Here's how the part is built. I have some questions about the finished solid (model axes, mm). A direction names the side the tool comes from. Round coordinates to 2 decimals unless told otherwise and drop trailing zeros. Loops run counter-clockwise (first coordinate to the right, second up) from the corner with the lowest first, then second, coordinate; pieces in that order, holes last. Notation, with made-up numbers: M -38,56 L 2,56 A10 cw 2,73 Z; hole C 19.5,79 d1. An arc over 180 degrees is marked long. Answer as CSV lines item,"result".
```python
from build123d import *

# Parameters (mm, degrees)
SKETCH_1_R          = 5.75
EXTRUDE_1_DEPTH     = 0.9
SKETCH_2_R          = 5.75
SKETCH_2_R_2        = 4.8
EXTRUDE_2_DEPTH     = 3.5
SKETCH_3_R          = 6.4
SKETCH_3_R_2        = 4.8
EXTRUDE_3_DEPTH     = 1.3
SKETCH_4_W          = 0.85
SKETCH_4_H          = 3.8
SKETCH_4_W_2        = 1.824882422
SKETCH_4_H_2        = 0.85
EXTRUDE_4_DEPTH     = 6.7
EXTRUDE_5_DEPTH     = 3.8
CUT_EXTRUDE_1_REACH = 10.3
EXTRUDE_6_DEPTH     = 4
FILLET1_R           = 0.2


with BuildPart() as part:
    # Эскиз1 → Бобышка-Вытянуть1 (new body)
    with BuildSketch(Plane(origin=(0, 0, 0), x_dir=(1, 0, 0), z_dir=(0, 1, 0))):
        Circle(SKETCH_1_R)
    extrude(amount=EXTRUDE_1_DEPTH)

    # Эскиз2 → Бобышка-Вытянуть2 (add)
    with BuildSketch(Plane(origin=(0, 0.9, 0), x_dir=(1, 0, 0), z_dir=(0, 1, 0))):
        Circle(SKETCH_2_R)
        Circle(SKETCH_2_R_2, mode=Mode.SUBTRACT)
    extrude(amount=EXTRUDE_2_DEPTH)

    # Эскиз3 → Бобышка-Вытянуть3 (add)
    with BuildSketch(Plane(origin=(0, 4.4, 0), x_dir=(1, 0, 0), z_dir=(0, 1, 0))):
        Circle(SKETCH_3_R)
        Circle(SKETCH_3_R_2, mode=Mode.SUBTRACT)
    extrude(amount=EXTRUDE_3_DEPTH)

    # Эскиз4 → Бобышка-Вытянуть4 (add)
    with BuildSketch(Plane(origin=(0, 0.9, 0), x_dir=(1, 0, 0), z_dir=(0, 1, 0))):
        with Locations((-2.325, 0)):
            Rectangle(SKETCH_4_W, SKETCH_4_H)
        with Locations((2.325, 0)):
            Rectangle(SKETCH_4_W, SKETCH_4_H)
        with Locations((0, 2.325)):
            Rectangle(SKETCH_4_W_2, SKETCH_4_H_2)
        with Locations((0, -2.325)):
            Rectangle(SKETCH_4_W_2, SKETCH_4_H_2)
    extrude(amount=EXTRUDE_4_DEPTH)

    # Эскиз5 → Бобышка-Вытянуть5 (add)
    with BuildSketch(Plane(origin=(0, 0, -1.9), x_dir=(-1, 0, 0), z_dir=(0, 0, -1))):
        Polygon((1.9, 6.3), (1.6, 6.6), (2.6, 7.6), align=None)
        Polygon((-1.9, 6.3), (-1.6, 6.6), (-2.6, 7.6), align=None)
    extrude(amount=-EXTRUDE_5_DEPTH)

    # Эскиз6 → Вырез-Вытянуть1 (cut, up to next)
    with BuildSketch(Plane(origin=(0, 0, -1.9), x_dir=(-1, 0, 0), z_dir=(0, 0, -1)), mode=Mode.PRIVATE) as cut_extrude_1_sk1:
        Polygon((1.9, 6.9), (2.6, 7.6), (1.9, 7.6), align=None)
    cut_extrude_1_tool1 = extrude(cut_extrude_1_sk1.sketch, amount=-CUT_EXTRUDE_1_REACH, mode=Mode.PRIVATE) & part.part
    add(cut_extrude_1_tool1.solids().sort_by_distance((-2.133333, 7.366667, -1.9))[0], mode=Mode.SUBTRACT)
    # Эскиз6 → Вырез-Вытянуть1 (cut, up to next)
    with BuildSketch(Plane(origin=(0, 0, -1.9), x_dir=(-1, 0, 0), z_dir=(0, 0, -1)), mode=Mode.PRIVATE) as cut_extrude_1_sk2:
        Polygon((-1.9, 6.9), (-2.6, 7.6), (-1.9, 7.6), align=None)
    cut_extrude_1_tool2 = extrude(cut_extrude_1_sk2.sketch, amount=-CUT_EXTRUDE_1_REACH, mode=Mode.PRIVATE) & part.part
    add(cut_extrude_1_tool2.solids().sort_by_distance((2.133333, 7.366667, -1.9))[0], mode=Mode.SUBTRACT)

    # Эскиз7 → Бобышка-Вытянуть6 (add)
    with BuildSketch(Plane(origin=(0, 0.9, 0), x_dir=(1, 0, 0), z_dir=(0, 1, 0))):
        with BuildLine():
            Line((-0.35, -2.75), (0.35, -2.75))
            Line((0.35, -2.75), (0.35, -4.787222577))
            ThreePointArc((0.35, -4.787222577), (0, -4.8), (-0.35, -4.787222577))
            Line((-0.35, -4.787222577), (-0.35, -2.75))
        make_face()
        with BuildLine():
            Line((4.787222577, -0.35), (2.75, -0.35))
            Line((2.75, -0.35), (2.75, 0.35))
            Line((2.75, 0.35), (4.787222577, 0.35))
            ThreePointArc((4.787222577, 0.35), (4.8, 0), (4.787222577, -0.35))
        make_face()
        with BuildLine():
            Line((0.35, 2.75), (0.35, 4.787222577))
            ThreePointArc((0.35, 4.787222577), (0, 4.8), (-0.35, 4.787222577))
            Line((-0.35, 4.787222577), (-0.35, 2.75))
            Line((-0.35, 2.75), (0.35, 2.75))
        make_face()
        with BuildLine():
            Line((-2.75, -0.35), (-4.787222577, -0.35))
            ThreePointArc((-4.787222577, -0.35), (-4.8, 0), (-4.787222577, 0.35))
            Line((-4.787222577, 0.35), (-2.75, 0.35))
            Line((-2.75, 0.35), (-2.75, -0.35))
        make_face()
    extrude(amount=EXTRUDE_6_DEPTH)

    # Fillet1
    fillet1_edges = [part.edges().sort_by_distance(p)[0] for p in [
        (-5.75, 0, 0),
    ]]
    fillet(fillet1_edges, radius=FILLET1_R)


solid = part.part
```
1. For P1, Ø0.7, axis at y = 3, z = -2.5, coming from the +X side; P2, Ø0.8, axis at x = -3.5, z = 0, coming from the +Y side; P3, Ø0.6, axis at x = -4, y = 2, coming from the -Z side, each with a flat end and sliding along its axis, tell me the tip position at first contact or that it passes through.
Evaluation:
P1,"stops at x = 5.33"
P2,"stops at y = 4.9"
P3,"stops at z = -4.4"
2. I want a section at C-C, the plane z = 0. Please give me the cut outline in (x, y).
Evaluation:
outline,"M -6.4,4.4 L -5.75,4.4 L -5.75,0.2 A0.2 ccw -5.55,0 L 5.55,0 A0.2 ccw 5.75,0.2 L 5.75,4.4 L 6.4,4.4 L 6.4,5.7 L 4.8,5.7 L 4.8,4.9 L 2.75,4.9 L 2.75,7.6 L 2.6,7.6 L 1.6,6.6 L 1.9,6.3 L 1.9,0.9 L -1.9,0.9 L -1.9,6.3 L -1.6,6.6 L -2.6,7.6 L -2.75,7.6 L -2.75,4.9 L -4.8,4.9 L -4.8,5.7 L -6.4,5.7 Z"
3. I want a section at B-B, the plane x = 0. Please give me the cut outline in (y, z), and give its area (3 significant figures).
Evaluation:
outline,"M 0,-5.55 A0.2 ccw 0.2,-5.75 L 4.4,-5.75 L 4.4,-6.4 L 5.7,-6.4 L 5.7,-4.8 L 4.9,-4.8 L 4.9,-2.75 L 7.6,-2.75 L 7.6,-1.9 L 0.9,-1.9 L 0.9,1.9 L 7.6,1.9 L 7.6,2.75 L 4.9,2.75 L 4.9,4.8 L 5.7,4.8 L 5.7,6.4 L 4.4,6.4 L 4.4,5.75 L 0.2,5.75 A0.2 ccw 0,5.55 Z"
area,"48.9 mm²"
4. Which directions (+Z, -Z, +X, -X, +Y, -Y) give clear straight access to the entire face, cutting with the end or side of a thin tool? Please do faces 1 (the flat face through (1.9, 4, 0)), 2 (the flat face through (0, 4, -1.9)), 3 (the flat face through (0, 7.6, 2.3)), 4 (the flat face through (-6, 4.4, -1)).
Evaluation:
face 1,"none"
face 2,"+Y"
face 3,"+Z, -Z, +X, -X, +Y"
face 4,"-Y"
5. If I drill on line 1 (Z direction, x = 0, y = 4.25); line 2 (X direction, y = 4.65, z = 0), over which ranges is the centre line in solid material (lowest first)? Write a range as [from, to].
Evaluation:
line 1,"z = [-5.75, -1.9], [1.9, 5.75]"
line 2,"x = [-6.4, -1.9], [1.9, 6.4]"
6. We'd pull the mould along X, two halves only. Please class faces 5 (the flat face through (0, 7.6, -2.3)), 6 (the flat face through (-0.35, 3, -4)), 7 (the cylindrical face through (-0.75, 2.27, -5.7)): pulls with the +X half, pulls with the -X half, needs draft (parallel to the pull), parting line crosses it, or undercut.
Evaluation:
face 5,"needs draft"
face 6,"undercut"
face 7,"parting line crosses it"
